Geometry: final body of the model. Coordinates: model frame, mm. A direction names the side the tool comes from. Coordinates: 2 decimals unless noted, no trailing zeros. Write each loop counter-clockwise with the first axis right and the second up, starting at its lowest first coordinate (ties: lowest second). Pieces come first, ordered by that corner, then holes. Notation, with made-up numbers: M 67,66.5 L 81,66.5 A21 ccw 81,93.5 Z; hole C 66,47 d6. An arc over 180 degrees is marked long. Write item = value, one per line. Start each with the question number.
Item 1: Pull-direction query (X, two-part tool) for faces 1 (the flat face through (-1.905, 10, 4)), 2 (the flat face through (13, 2, 7.62)), 3 (the flat face through (1.905, -13, 8)), 4 (the cylindrical face through (14.22, -0.29, 8.25)); classes: +X half, -X half, draft (parallel to the pull), parting line (faces both ways), or undercut.
Item 2: First-contact query: pin 1 Ø1.8 at (y, z) = (-8, 6) entering from -X; pin 2 Ø3 at (x, y) = (11, 11) entering from -Z; pin 3 Ø0.6 at (y, z) = (-13, 8.5) entering from -X; pin 4 Ø1 at (x, y) = (-5, -1) entering from -Z. Flat tips, straight axial feed; report the tip coordinate or a pass-through.
Item 3: Reachability of faces 5 (the flat face through (1.905, 10, 4)), 6 (the cylindrical face through (-7.11, 0.13, 4.38)), 7 (the flat face through (-13, 0, 7.62)), 8 (the flat face through (-1.905, -13, 8)) from +Z, -Z, +X, -X, +Y, -Y: full face, straight path, thin tool, end or side. Return the list, or none.
Item 4: Section A-A on y = 0. Output: boundary loops of the cut face in (x, z).
Item 5: Section B-B on z = 8.25. Output: boundary loops of the cut face in (x, y) (3 decimals).
Item 6: Ray query, L1, parallel to Z at x = -6.5, y = 11.5; L2, parallel to Y at x = -6.25, z = 0.75; L3, parallel to Y at x = 0.25, z = 2.75. Return the intervals inside material, ascending. Write a range as [from, to].
Item 7: Section C-C on x = -3. Output: boundary loops of the cut face in (y, z).
Item 8: Section D-D on x = 0. Output: boundary loops of the cut face in (y, z), plus the area to 3 significant figures.
from build123d import *

# Parameters (mm, degrees)
SKETCH1_R           = 12.7
SKETCH1_R_2         = 7.112
BOSS_EXTRUDE1_DEPTH = 7.62
SKETCH2_R           = 14.224
SKETCH2_R_2         = 7.112
BOSS_EXTRUDE2_DEPTH = 1.27
CUT_EXTRUDE1_DEPTH  = 9.89
CUT_EXTRUDE2_DEPTH  = 2.27
FILLET1_R           = 0.762


with BuildPart() as part:
    # Sketch1 → Boss-Extrude1 (new body)
    with BuildSketch(Plane.XY):
        Circle(SKETCH1_R)
        Circle(SKETCH1_R_2, mode=Mode.SUBTRACT)
    extrude(amount=BOSS_EXTRUDE1_DEPTH)

    # Sketch2 → Boss-Extrude2 (add)
    with BuildSketch(Plane.XY.offset(7.62)):
        Circle(SKETCH2_R)
        Circle(SKETCH2_R_2, mode=Mode.SUBTRACT)
    extrude(amount=BOSS_EXTRUDE2_DEPTH)

    # Sketch3 → Cut-Extrude1 (cut, through all)
    with BuildSketch(Plane(origin=(0, 0, 0), x_dir=(-1, 0, 0), z_dir=(0, 0, -1))):
        with BuildLine():
            Line((-1.905, 14.224), (1.905, 14.224))
            Line((1.905, 14.224), (1.905, -11.141309797))
            ThreePointArc((1.905, -11.141309797), (0, -11.303), (-1.905, -11.141309797))
            Line((-1.905, -11.141309797), (-1.905, 14.224))
        make_face()
    extrude(amount=-CUT_EXTRUDE1_DEPTH, mode=Mode.SUBTRACT)

    # Sketch4 → Cut-Extrude2 (cut, through all)
    with BuildSketch(Plane(origin=(0, 0, 7.62), x_dir=(-1, 0, 0), z_dir=(0, 0, -1))):
        with BuildLine():
            Line((-1.905, -14.224), (-1.905, -12.556312158))
            ThreePointArc((-1.905, -12.556312158), (0, -12.7), (1.905, -12.556312158))
            Line((1.905, -12.556312158), (1.905, -14.224))
            Line((1.905, -14.224), (-1.905, -14.224))
        make_face()
    extrude(amount=-CUT_EXTRUDE2_DEPTH, mode=Mode.SUBTRACT)

    # Fillet1
    fillet1_edges = [part.edges().sort_by_distance(p)[0] for p in [
        (1.905, -11.141309797, 4.445),
        (-1.905, -11.141309797, 4.445),
    ]]
    fillet(fillet1_edges, radius=FILLET1_R)


solid = part.part
Responses:
q1.face_1 = undercut
q1.face_2 = draft
q1.face_3 = undercut
q1.face_4 = +X half
q2.pin_1 = -10.53
q2.pin_2 = 7.62
q2.pin_3 = -6.41
q2.pin_4 = through
q3.face_5 = +Z, -Z, +Y
q3.face_6 = +Z, -Z
q3.face_7 = -Z, -X
q3.face_8 = +Z, -Z, -Y
q4.outline = M -14.22,7.62 L -12.7,7.62 L -12.7,0 L -7.11,0 L -7.11,8.89 L -14.22,8.89 Z; M 7.11,0 L 12.7,0 L 12.7,7.62 L 14.22,7.62 L 14.22,8.89 L 7.11,8.89 Z
q5.outline = M -1.905,-14.096 L -1.905,-12.556 A12.7 ccw 1.905,-12.556 L 1.905,-14.096 A14.224 ccw 1.905,14.096 L 1.905,6.852 A7.112 cw 1.905,-6.852 L 1.905,-10.479 A0.762 cw 1.226,-11.236 A11.303 cw -1.226,-11.236 A0.762 cw -1.905,-10.479 L -1.905,-6.852 A7.112 cw -1.905,6.852 L -1.905,14.096 A14.224 ccw Z
q6.L1 = [7.62, 8.89]
q6.L2 = [-11.06, -3.39], [3.39, 11.06]
q6.L3 = [-12.7, -11.3]
q7.outline = M -13.9,7.62 L -12.34,7.62 L -12.34,0 L -6.45,0 L -6.45,8.89 L -13.9,8.89 Z; M 6.45,0 L 12.34,0 L 12.34,7.62 L 13.9,7.62 L 13.9,8.89 L 6.45,8.89 Z
q8.outline = M -12.7,0 L -11.3,0 L -11.3,8.89 L -12.7,8.89 Z
q8.area = 12.4 mm²
